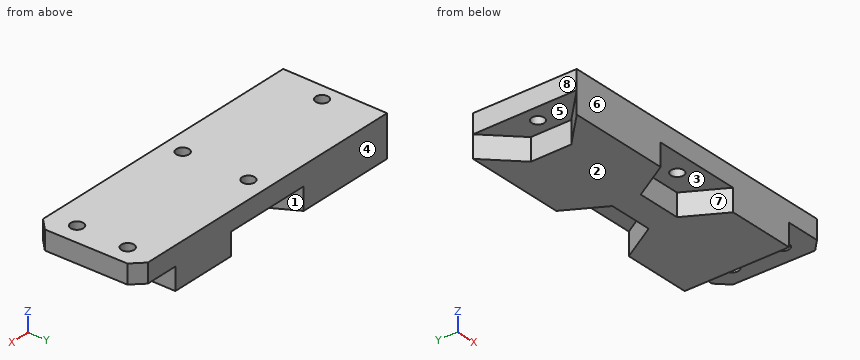
```python
from build123d import *

# Parameters (mm, degrees)
BOSS_EXTRUDE1_DEPTH = 6
BOSS_EXTRUDE2_DEPTH = 7
CUT_EXTRUDE1_REACH  = 143.419
SKETCH3_R           = 2
CUT_EXTRUDE2_START  = -13
CUT_EXTRUDE2_DEPTH  = 7
CUT_EXTRUDE3_REACH  = 142.994
SKETCH5_R           = 2


with BuildPart() as part:
    # Sketch1 → Boss-Extrude1 (new body)
    with BuildSketch(Plane.XY):
        Polygon((44.15, 19.080039823), (135.5692396, 19.080039823), (139.116658887, 15.519822908), (139.521129618, -10.195951693), (135.999179687, -13.705241552), (44.15, -13.705241552), align=None)
    extrude(amount=BOSS_EXTRUDE1_DEPTH)

    # Sketch2 → Boss-Extrude2 (add)
    with BuildSketch(Plane(origin=(0, 0, 0), x_dir=(-1, 0, 0), z_dir=(0, 0, -1))):
        Polygon((-125.069457212, 19.080039823), (-125.284105894, -13.705241552), (-44.15, -13.705241552), (-54.15, -3.705241552), (-54.15, 9.080039823), (-44.15, 19.080039823), align=None)
    extrude(amount=BOSS_EXTRUDE2_DEPTH)

    # Sketch3 → Cut-Extrude1 (cut, up to next)
    with BuildSketch(Plane(origin=(0, 0, -7), x_dir=(-1, 0, 0), z_dir=(0, 0, -1)), mode=Mode.PRIVATE) as cut_extrude1_sk1:
        with Locations((-133.124576169, 10.687399136)):
            Circle(SKETCH3_R)
    cut_extrude1_tool1 = extrude(cut_extrude1_sk1.sketch, amount=-CUT_EXTRUDE1_REACH, mode=Mode.PRIVATE) & part.part
    # Sketch3 → Cut-Extrude1 (cut, up to next)
    with BuildSketch(Plane(origin=(0, 0, -7), x_dir=(-1, 0, 0), z_dir=(0, 0, -1)), mode=Mode.PRIVATE) as cut_extrude1_sk2:
        with Locations((-133.124576169, -5.312600864)):
            Circle(SKETCH3_R)
    cut_extrude1_tool2 = extrude(cut_extrude1_sk2.sketch, amount=-CUT_EXTRUDE1_REACH, mode=Mode.PRIVATE) & part.part
    # Sketch3 → Cut-Extrude1 (cut, up to next)
    with BuildSketch(Plane(origin=(0, 0, -7), x_dir=(-1, 0, 0), z_dir=(0, 0, -1)), mode=Mode.PRIVATE) as cut_extrude1_sk3:
        with Locations((-49.15, 2.687399136)):
            Circle(SKETCH3_R)
    cut_extrude1_tool3 = extrude(cut_extrude1_sk3.sketch, amount=-CUT_EXTRUDE1_REACH, mode=Mode.PRIVATE) & part.part
    add(cut_extrude1_tool1.solids().sort_by_distance((133.124576, 10.687399, -7))[0], mode=Mode.SUBTRACT)
    add(cut_extrude1_tool2.solids().sort_by_distance((133.124576, -5.312601, -7))[0], mode=Mode.SUBTRACT)
    add(cut_extrude1_tool3.solids().sort_by_distance((49.15, 2.687399, -7))[0], mode=Mode.SUBTRACT)

    # Sketch4 → Cut-Extrude2 (cut)
    with BuildSketch(Plane.XY.offset(6).offset(CUT_EXTRUDE2_START)):
        Polygon((76.218183383, -13.705241552), (83.146386613, -25.705241552), (97.002793074, -25.705241552), (103.930996304, -13.705241552), (97.002793074, -1.705241552), (83.146386613, -1.705241552), align=None)
        Polygon((76.003213339, 19.080039823), (82.93141657, 7.080039823), (96.78782303, 7.080039823), (103.71602626, 19.080039823), (96.78782303, 31.080039823), (82.93141657, 31.080039823), align=None)
    extrude(amount=CUT_EXTRUDE2_DEPTH, mode=Mode.SUBTRACT)

    # Sketch5 → Cut-Extrude3 (cut, up to next)
    with BuildSketch(Plane(origin=(0, 0, 0), x_dir=(-1, 0, 0), z_dir=(0, 0, -1)), mode=Mode.PRIVATE) as cut_extrude3_sk1:
        with Locations((-89.8596198, 13.080039823)):
            Circle(SKETCH5_R)
    cut_extrude3_tool1 = extrude(cut_extrude3_sk1.sketch, amount=-CUT_EXTRUDE3_REACH, mode=Mode.PRIVATE) & part.part
    # Sketch5 → Cut-Extrude3 (cut, up to next)
    with BuildSketch(Plane(origin=(0, 0, 0), x_dir=(-1, 0, 0), z_dir=(0, 0, -1)), mode=Mode.PRIVATE) as cut_extrude3_sk2:
        with Locations((-89.8596198, -7.705241552)):
            Circle(SKETCH5_R)
    cut_extrude3_tool2 = extrude(cut_extrude3_sk2.sketch, amount=-CUT_EXTRUDE3_REACH, mode=Mode.PRIVATE) & part.part
    add(cut_extrude3_tool1.solids().sort_by_distance((89.85962, 13.08004, 0))[0], mode=Mode.SUBTRACT)
    add(cut_extrude3_tool2.solids().sort_by_distance((89.85962, -7.705242, 0))[0], mode=Mode.SUBTRACT)


solid = part.part
```
Here's how the part is built. I have some questions about the finished solid (model axes, mm). Face numbers are marked on the shaded views. A direction names the side the tool comes from. Coordinates: 2 decimals unless noted, no trailing zeros. Order: outer loops, then holes, each group sorted by start corner. A loop starts at its lowest first (then second) coordinate and runs counter-clockwise, first axis right, second up. Notation, with made-up numbers: (-26, -17.75) - (-20, -17.75) arc R25 ccw to (-20, 5.25) - close; hole circle Ø4 at (71.25, 26). An arc over 180 degrees is marked (long way). One line per question, with ' | ' between items. Start each with the question number.
1. If we section it at A-A (z = -5.25): Write out the boundary of the cut face in (x, y).
2. Which directions (+Z, -Z, +X, -X, +Y, -Y) give clear straight access to the entire face, cutting with the end or side of a thin tool? Please do the marked faces 1, 2, 3, 4 and 5.
3. I'm going to push flat-ended pins straight in: pin 1 Ø3.5 at (y, z) = (5, -5) entering from -X; pin 2 Ø1.5 at (y, z) = (9.5, -1) entering from +X; pin 3 Ø5 at (x, y) = (133.12, -5.31) entering from -Z; pin 4 Ø2.5 at (x, y) = (133.12, 10.69) entering from +Z. Where does each tip first touch, or does it pass through?
4. If we mould it in two halves opening along X, with no side actions, what happens to the marked faces 6, 7 and 8? For each: released by +X, released by -X, zero draft, split by the parting line, or undercut.
5. Please list where these lines run through material, in increasing order: line 1 along Z through (x, y) = (83, 8.5); line 2 along Y through (x, z) = (49.15, 3); line 3 along X through (y, z) = (-7, 0.25). Write a range as [from, to].
6. If we section it at B-B (x = 49.15): Write out the boundary of the cut face in (y, z), and give its area (3 significant figures).
7. If we section it at C-C (z = 1.25): Write out the boundary of the cut face in (x, y).
Model answer:
1) outline: (44.15, -13.71) - (76.22, -13.71) - (83.15, -1.71) - (97, -1.71) - (103.93, -13.71) - (125.28, -13.71) - (125.07, 19.08) - (103.72, 19.08) - (96.79, 7.08) - (82.93, 7.08) - (76, 19.08) - (44.15, 19.08) - (54.15, 9.08) - (54.15, -3.71) - close
2) face 1: -Z, +Y | face 2: -Z, +X, -X, +Y, -Y | face 3: -Z, -Y | face 4: +Z, -Z, +X, -X, +Y | face 5: -Z, -X
3) pin 1: stops at x = 54.15 | pin 2: stops at x = 125.14 | pin 3: stops at z = 0 | pin 4: passes through
4) face 6: zero draft | face 7: undercut | face 8: released by -X
5) line 1: z = [0, 6] | line 2: y = [-13.71, 0.69], [4.69, 19.08] | line 3: x = [44.15, 87.99], [91.73, 132.05], [134.2, 139.47]
6) outline: (-13.71, -7) - (-8.71, -7) - (-8.71, 0) - (0.69, 0) - (0.69, 6) - (-13.71, 6) - close; (4.69, 0) - (14.08, 0) - (14.08, -7) - (19.08, -7) - (19.08, 6) - (4.69, 6) - close | area: 243 mm²
7) outline: (44.15, -13.71) - (136, -13.71) - (139.52, -10.2) - (139.12, 15.52) - (135.57, 19.08) - (44.15, 19.08) - close; hole circle Ø4 at (49.15, 2.69); hole circle Ø4 at (89.86, -7.71); hole circle Ø4 at (89.86, 13.08); hole circle Ø4 at (133.12, -5.31); hole circle Ø4 at (133.12, 10.69)
